```python
from build123d import *

# Parameters (mm, degrees)
SKETCH1_R                  = 2.54
SKETCH1_R_2                = 9.525
BOSS_EXTRUDE1_DEPTH        = 4.7625
CONVERT_SOLID1_OUTLINE_R   = 2.54
CONVERT_SOLID1_OUTLINE_R_2 = 9.525
CONVERT_SOLID1_DEPTH       = 1.5875


# Read off the part's stored shape, not the designer's step: Convert-Solid1
with BuildPart() as part:
    # Sketch1 → Boss-Extrude1 (new body)
    with BuildSketch(Plane(origin=(0, 0, 0), x_dir=(0, 0, -1), z_dir=(1, 0, 0))):
        with BuildLine():
            Line((517.497208961, 116.457539853), (677.757490375, 101.56617639))
            ThreePointArc((677.757490375, 101.56617639), (682.684377991, 99.111706327), (684.672478048, 93.978860817))
            Line((684.672478048, 93.978860817), (684.672478048, 43.274288567))
            ThreePointArc((684.672478048, 43.274288567), (680.952734169, 34.294032445), (671.972478048, 30.574288567))
            Line((671.972478048, 30.574288567), (519.572478048, 30.574288567))
            ThreePointArc((519.572478048, 30.574288567), (510.592221927, 34.294032445), (506.872478048, 43.274288567))
            Line((506.872478048, 43.274288567), (506.872478048, 106.774288567))
            ThreePointArc((506.872478048, 106.774288567), (510.046689227, 113.961956173), (517.497208961, 116.457539853))
        make_face()
        with Locations(Location((515.911244675, 107.527203865, 0), (0, 0, 180))):
            Circle(SKETCH1_R, mode=Mode.SUBTRACT)
        with Locations(Location((550.052478048, 75.024288567, 0), (0, 0, 180))):
            Circle(SKETCH1_R_2, mode=Mode.SUBTRACT)
        with Locations(Location((595.772478048, 75.024288567, 0), (0, 0, 180))):
            Circle(SKETCH1_R_2, mode=Mode.SUBTRACT)
        with Locations(Location((605.297478048, 51.47785837, 0), (0, 0, 180))):
            Circle(SKETCH1_R, mode=Mode.SUBTRACT)
        with Locations(Location((586.247478048, 98.570718763, 0), (0, 0, 180))):
            Circle(SKETCH1_R, mode=Mode.SUBTRACT)
        with Locations(Location((641.492478048, 75.024288567, 0), (0, 0, 180))):
            Circle(SKETCH1_R_2, mode=Mode.SUBTRACT)
        with Locations(Location((605.297478048, 36.924288567, 0), (0, 0, 180))):
            Circle(SKETCH1_R, mode=Mode.SUBTRACT)
        with Locations(Location((586.247478048, 36.924288567, 0), (0, 0, 180))):
            Circle(SKETCH1_R, mode=Mode.SUBTRACT)
        with Locations(Location((519.572478048, 43.274288567, 0), (0, 0, 180))):
            Circle(SKETCH1_R, mode=Mode.SUBTRACT)
        with Locations(Location((671.972478048, 43.274288567, 0), (0, 0, 180))):
            Circle(SKETCH1_R, mode=Mode.SUBTRACT)
    extrude(amount=BOSS_EXTRUDE1_DEPTH)

    # Convert-Solid1 outline → Convert-Solid1 (cut)
    with BuildSketch(Plane.YZ):
        with BuildLine():
            ThreePointArc((116.457539853, -517.497208961), (113.961956173, -510.046689227), (106.774288567, -506.872478048))
            Line((106.774288567, -506.872478048), (43.274288567, -506.872478048))
            ThreePointArc((43.274288567, -506.872478048), (34.294032446, -510.592221927), (30.574288567, -519.572478048))
            Line((30.574288567, -519.572478048), (30.574288567, -671.972478048))
            ThreePointArc((30.574288567, -671.972478048), (34.294032445, -680.952734169), (43.274288567, -684.672478048))
            Line((43.274288567, -684.672478048), (93.978860817, -684.672478048))
            ThreePointArc((93.978860817, -684.672478048), (99.111706327, -682.684377991), (101.56617639, -677.757490375))
            Line((101.56617639, -677.757490375), (116.457539853, -517.497208961))
        make_face()
        with Locations((43.274288567, -671.972478048)):
            Circle(CONVERT_SOLID1_OUTLINE_R, mode=Mode.SUBTRACT)
        with Locations((36.924288567, -605.297478048)):
            Circle(CONVERT_SOLID1_OUTLINE_R, mode=Mode.SUBTRACT)
        with Locations((51.47785837, -605.297478048)):
            Circle(CONVERT_SOLID1_OUTLINE_R, mode=Mode.SUBTRACT)
        with Locations((75.024288567, -641.492478048)):
            Circle(CONVERT_SOLID1_OUTLINE_R_2, mode=Mode.SUBTRACT)
        with Locations((75.024288567, -595.772478048)):
            Circle(CONVERT_SOLID1_OUTLINE_R_2, mode=Mode.SUBTRACT)
        with Locations((36.924288567, -586.247478048)):
            Circle(CONVERT_SOLID1_OUTLINE_R, mode=Mode.SUBTRACT)
        with Locations((43.274288567, -519.572478048)):
            Circle(CONVERT_SOLID1_OUTLINE_R, mode=Mode.SUBTRACT)
        with Locations((98.570718763, -586.247478048)):
            Circle(CONVERT_SOLID1_OUTLINE_R, mode=Mode.SUBTRACT)
        with Locations((75.024288567, -550.052478048)):
            Circle(CONVERT_SOLID1_OUTLINE_R_2, mode=Mode.SUBTRACT)
        with Locations((107.527203865, -515.911244675)):
            Circle(CONVERT_SOLID1_OUTLINE_R, mode=Mode.SUBTRACT)
    extrude(amount=CONVERT_SOLID1_DEPTH, mode=Mode.SUBTRACT)


solid = part.part
```
The model under review builds one solid part; all positions refer to its coordinate system, in mm. Give positions to 0.01 mm unless a question says otherwise; leave off trailing zeros. Write each loop counter-clockwise with the first axis right and the second up, starting at its lowest first coordinate (ties: lowest second). Pieces come first, ordered by that corner, then holes. Notation, with made-up numbers: M -3.75,-21.75 L 25.25,-21.75 A18 ccw 25.25,-9.75 Z; hole C 0.5,-14 d3. An arc over 180 degrees is marked long. Write each question's results on one line, items separated by ' | '. Start each with the question number.
1. We need section C-C (y = 82.5). Write out the cut boundary in (x, z), and give its area (3 significant figures).
2. For probe 1 along Z at (x, y) = (3.7, 73); probe 2 along Z at (x, y) = (3.9, 68); probe 3 along Z at (x, y) = (2.8, 45), list the stretches that pass through material, from the lowest coordinate up. Write a range as [from, to].
3. We need section B-B (x = 3.9). Count the separate pieces of the cut face and the enclosed holes in it, and give its area (3 significant figures).
4. Insertion check: pin 1 Ø4.5 at (y, z) = (36.92, -605.3) entering from +X. The pin has a flat end and moves straight along its axis. Give the tip position at first contact, or say it passes through.
5. We need section D-D (z = -597). Write out the cut boundary in (x, y), and give its area (3 significant figures).
6. Mouldability with a two-part tool opening along Z and no side actions: class faces 1 (the cylindrical face through (3.15, 34.2, -510.69)), 2 (the cylindrical face through (3.15, 42.51, -517.15)), 3 (the cylindrical face through (3.15, 34.39, -681.05)) as released by +Z, released by -Z, zero draft, split by the parting line, or undercut.
7. We need section A-A (z = -635). Write out the cut boundary in (x, y).
Results found:
1) outline: M 1.59,-684.67 L 4.76,-684.67 L 4.76,-647.39 L 1.59,-647.39 Z; M 1.59,-635.59 L 4.76,-635.59 L 4.76,-601.67 L 1.59,-601.67 Z; M 1.59,-589.87 L 4.76,-589.87 L 4.76,-555.95 L 1.59,-555.95 Z; M 1.59,-544.15 L 4.76,-544.15 L 4.76,-506.87 L 1.59,-506.87 Z | area: 452 mm^2
2) probe 1: z = [-684.67, -650.8], [-632.19, -605.08], [-586.47, -559.36], [-540.75, -506.87] | probe 2: z = [-684.67, -647.93], [-635.06, -602.21], [-589.34, -556.49], [-543.62, -506.87] | probe 3: z = [-684.67, -673.84], [-670.11, -521.44], [-517.71, -506.87]
3) separate pieces: 1 | enclosed holes: 10 | area: 12,900 mm^2
4) pin 1: passes through
5) outline: M 1.59,30.57 L 4.76,30.57 L 4.76,65.58 L 1.59,65.58 Z; M 1.59,84.47 L 4.76,84.47 L 4.76,109.07 L 1.59,109.07 Z | area: 189 mm^2
6) face 1: released by +Z | face 2: undercut | face 3: released by -Z
7) outline: M 1.59,30.57 L 4.76,30.57 L 4.76,68.05 L 1.59,68.05 Z; M 1.59,81.99 L 4.76,81.99 L 4.76,105.54 L 1.59,105.54 Z
